Here's how the part is built. I have some questions about the finished solid (model axes, mm). Round coordinates to 2 decimals unless told otherwise and drop trailing zeros. Loops run counter-clockwise (first coordinate to the right, second up) from the corner with the lowest first, then second, coordinate; pieces in that order, holes last. Notation, with made-up numbers: M 56,15.5 L 72,15.5 A8 cw 72,20.5 Z; hole C 64.25,37 d11. An arc over 180 degrees is marked long. Answer as a JSON object with one key per item and string values.
from build123d import *

# Parameters (mm, degrees)
ESQUISSE1_R        = 2
BOSS_EXTRU_1_DEPTH = 2
BOSS_EXTRU_2_DEPTH = 22
CHANFREIN1_SIZE    = 1


with BuildPart() as part:
    # Esquisse1 → Boss.-Extru.1 (new body)
    with BuildSketch(Plane.XY):
        with BuildLine():
            Line((8.5, 0), (43.5, 0))
            ThreePointArc((43.5, 0), (49.51040764, -2.48959236), (52, -8.5))
            Line((52, -8.5), (52, -9.5))
            ThreePointArc((52, -9.5), (49.51040764, -15.51040764), (43.5, -18))
            Line((43.5, -18), (8.5, -18))
            ThreePointArc((8.5, -18), (2.48959236, -15.51040764), (0, -9.5))
            Line((0, -9.5), (0, -8.5))
            ThreePointArc((0, -8.5), (2.48959236, -2.48959236), (8.5, 0))
        make_face()
        with Locations((10, -9)):
            Circle(ESQUISSE1_R, mode=Mode.SUBTRACT)
        with Locations((42, -9)):
            Circle(ESQUISSE1_R, mode=Mode.SUBTRACT)
    extrude(amount=BOSS_EXTRU_1_DEPTH)

    # Esquisse2 → Boss.-Extru.2 (add)
    with BuildSketch(Plane(origin=(0, 0, 0), x_dir=(-1, 0, 0), z_dir=(0, 0, -1))):
        with BuildLine():
            ThreePointArc((-35, -9), (-32.363961031, -15.363961031), (-26, -18))
            Line((-26, -18), (-26, -9))
            Line((-26, -9), (-35, -9))
        make_face()
        with BuildLine():
            Line((-26, -9), (-26, -18))
            ThreePointArc((-26, -18), (-19.636038969, -15.363961031), (-17, -9))
            Line((-17, -9), (-26, -9))
        make_face()
        with BuildLine():
            Line((-35, -9), (-26, -9))
            Line((-26, -9), (-26, 0))
            ThreePointArc((-26, 0), (-32.363961031, -2.636038969), (-35, -9))
        make_face()
        with BuildLine():
            Line((-26, 0), (-26, -9))
            Line((-26, -9), (-17, -9))
            ThreePointArc((-17, -9), (-19.636038969, -2.636038969), (-26, 0))
        make_face()
    extrude(amount=BOSS_EXTRU_2_DEPTH)

    # Chanfrein1
    chanfrein1_edges = [part.edges().sort_by_distance(p)[0] for p in [
        (8, -9, 2),
        (40, -9, 2),
    ]]
    chamfer(chanfrein1_edges, length=CHANFREIN1_SIZE)


solid = part.part
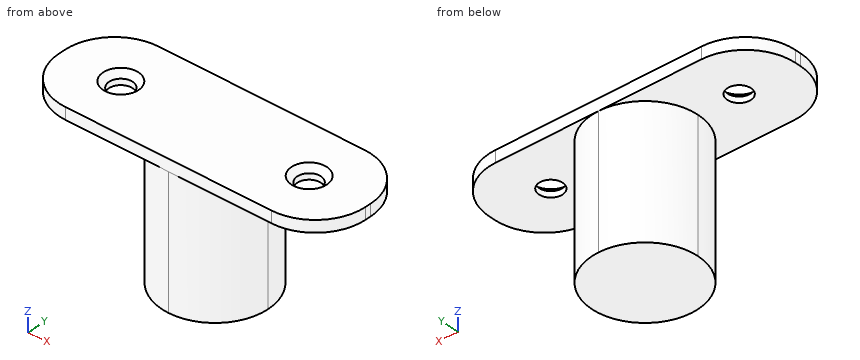
Item 1: For P1, Ø1.5, axis at y = -3, z = -11, coming from the +X side; P2, Ø6.5, axis at x = 10, y = -9, coming from the +Z side; P3, Ø1, axis at x = 6, y = -4, coming from the -Z side; P4, Ø1.5, axis at y = -14.5, z = -4, coming from the +X side, each with a flat end and sliding along its axis, tell me the tip position at first contact or that it passes through.
Solution:
{"P1": "stops at x = 33.31", "P2": "stops at z = 2", "P3": "stops at z = 0", "P4": "stops at x = 33.64"}
Item 2: I want a section at C-C on x = 31. List the corners of the cut face in (y, z) for me.
Solution:
{"outline": "M -18,0 L -16.48,0 L -16.48,-22 L -1.52,-22 L -1.52,0 L 0,0 L 0,2 L -18,2 Z"}
Item 3: I want a section at D-D on y = -7.75. Count the separate pieces of the cut face and the enclosed holes in it, plus the area to 3 significant figures.
Solution:
{"separate pieces": "3", "enclosed holes": "0", "area": "481 mm2"}
Item 4: I want a section at A-A on x = 10. List the corners of the cut face in (y, z) for me, plus the area to 3 significant figures.
Solution:
{"outline": "M -18,0 L -11,0 L -11,1 L -12,2 L -18,2 Z; M -7,0 L 0,0 L 0,2 L -6,2 L -7,1 Z", "area": "27.0 mm2"}
Item 5: If I drill on L1, parallel to Y at x = 42, z = 0.45; L2, parallel to Z at x = 17, y = -5.25; L3, parallel to X at y = -8.5, z = -6, over which ranges is the centre line in solid material (lowest first)? Write a range as from..to.
Solution:
{"L1": "y = -18..-11, -7..0", "L2": "z = 0..2", "L3": "x = 17.01..34.99"}
Item 6: I want a section at B-B on y = -1.75. List the corners of the cut face in (x, z) for me, plus the area to 3 significant figures.
Solution:
{"outline": "M 3.33,0 L 20.67,0 L 20.67,-22 L 31.33,-22 L 31.33,0 L 48.67,0 L 48.67,2 L 3.33,2 Z", "area": "325 mm2"}
